Can you work these out from the model? Positions are in its coordinate system, mm. Coordinates: 2 decimals unless noted, no trailing zeros. Write each loop counter-clockwise with the first axis right and the second up, starting at its lowest first coordinate (ties: lowest second). Pieces come first, ordered by that corner, then holes. Notation, with made-up numbers: (-29, 65) - (0, 65) arc R14 ccw to (0, 72) - close; hole circle Ø3 at (66, 59). An arc over 180 degrees is marked (long way). Use one line per item in the form item = value. Start each with the question number.
(1) If we section it at A-A on x = 3.5: Please give me the cut outline in (y, z) (3 decimals).
(2) If we section it at B-B on z = 1478: Please give me the cut outline in (x, y) (3 decimals), then the cut area to 3 significant figures.
(3) If I drill on probe 1 along Y at (x, z) = (-1, 101.5) (3 decimals); probe 2 along X at (y, z) = (10.5, 1108.5), over which ranges is the centre line in solid material (lowest first)? Write a range as from..to.
Autodesk Inventor part; units mm, degrees
ref_plane "Start Plane" through (0, 0, 0) normal (0, 0, 1) x (1, 0, 0)
ref_plane "End Plane" through (0, 0, 1700) normal (0, 0, 1) x (1, 0, 0)
ref_plane "YZ Plane" through (0, 0, 0) normal (1, 0, 0) x (0, 1, 0)
ref_plane "Start Plane" through (0, 0, 0) normal (0, 0, 1) x (1, 0, 0)
ref_plane "End Plane" through (0, 0, 1700) normal (0, 0, 1) x (1, 0, 0)
sketch "Sketch" plane through (0, 0, 0) normal (0, 0, 1) x (1, 0, 0)
  line L0 (-15.875, -9.525) -> (-15.875, 9.525)
  line L1 (-9.525, 15.875) -> (9.525, 15.875)
  line L2 (15.875, 9.525) -> (15.875, -9.525)
  line L3 (9.525, -15.875) -> (-9.525, -15.875)
  arc A0 (-15.875, -9.525) -> (-9.525, -15.875) centre (-9.525, -9.525) ccw
  arc A1 (-9.525, 15.875) -> (-15.875, 9.525) centre (-9.525, 9.525) ccw
  arc A2 (15.875, 9.525) -> (9.525, 15.875) centre (9.525, 9.525) ccw
  arc A3 (9.525, -15.875) -> (15.875, -9.525) centre (9.525, -9.525) ccw
  arc A4 (-9.525, 12.7) -> (-12.7, 9.525) centre (-9.525, 9.525) ccw
  line L4 (-9.525, 12.7) -> (9.525, 12.7)
  arc A5 (12.7, 9.525) -> (9.525, 12.7) centre (9.525, 9.525) ccw
  line L5 (12.7, 9.525) -> (12.7, -9.525)
  arc A6 (9.525, -12.7) -> (12.7, -9.525) centre (9.525, -9.525) ccw
  line L6 (9.525, -12.7) -> (-9.525, -12.7)
  arc A7 (-12.7, -9.525) -> (-9.525, -12.7) centre (-9.525, -9.525) ccw
  line L7 (-12.7, -9.525) -> (-12.7, 9.525)
  line L8 (0, 24.0662) -> (0, -24.0662) construction
  line L9 (-24.0662, 0) -> (24.0662, 0) construction
  dimension "d10" = 31.75
  dimension "d11" = 31.75
  dimension "d12" = 3.175
  dimension "d15" = 15.875
  dimension "d16" = 15.875
  dimension "d17" = 6.35
extrude "Body" add sketch "Sketch" along normal up to surface (1700 mm away) from surface at 0
sketch "Sketch3" plane through (0, 0, 0) normal (0, 0, 1) x (1, 0, 0)
  line L0 (0, 0) -> (10, 0)
ref_plane "Work Plane3" through (0, 0, 0) normal (0, -1, 0) x (1, 0, 0)
sketch "Sketch5" plane through (-15.875, 9.525, 0) normal (-1, 0, 0) x (0, 0, 1)
  line L0 (309.525, 3.175) -> (290.475, 3.175)
  arc A0 (312.7, 0) -> (309.525, 3.175) centre (309.525, 0) ccw
  line L1 (312.7, -19.05) -> (312.7, 0)
  arc A1 (309.525, -22.225) -> (312.7, -19.05) centre (309.525, -19.05) ccw
  line L2 (290.475, -22.225) -> (309.525, -22.225)
  arc A2 (287.3, -19.05) -> (290.475, -22.225) centre (290.475, -19.05) ccw
  line L3 (287.3, 0) -> (287.3, -19.05)
  arc A3 (290.475, 3.175) -> (287.3, 0) centre (290.475, 0) ccw
  line L4 (284.125, -19.05) -> (284.125, 0)
  arc A4 (284.125, -19.05) -> (290.475, -25.4) centre (290.475, -19.05) ccw
  line L5 (309.525, -25.4) -> (290.475, -25.4)
  arc A5 (309.525, -25.4) -> (315.875, -19.05) centre (309.525, -19.05) ccw
  line L6 (315.875, 0) -> (315.875, -19.05)
  arc A6 (315.875, 0) -> (309.525, 6.35) centre (309.525, 0) ccw
  line L7 (290.475, 6.35) -> (309.525, 6.35)
  arc A7 (290.475, 6.35) -> (284.125, 0) centre (290.475, 0) ccw
  circle A8 centre (293.65, -9.525) radius 4
  line L8 (300, -22.225) -> (300, 3.175)
  line L9 (293.65, -3.1741) -> (299.15, -6.3496)
  line L10 (299.15, -6.3496) -> (299.15, -12.7004)
  line L11 (299.15, -12.7004) -> (293.65, -15.8759)
  line L12 (293.65, -15.8759) -> (288.15, -12.7004)
  line L13 (288.15, -12.7004) -> (288.15, -6.3496)
  line L14 (288.15, -6.3496) -> (293.65, -3.1741)
  circle A9 centre (306.35, -9.525) radius 4
  line L15 (306.35, -3.1741) -> (300.85, -6.3496)
  line L16 (300.85, -6.3496) -> (300.85, -12.7004)
  line L17 (300.85, -12.7004) -> (306.35, -15.8759)
  line L18 (306.35, -15.8759) -> (311.85, -12.7004)
  line L19 (311.85, -12.7004) -> (311.85, -6.3496)
  line L20 (311.85, -6.3496) -> (306.35, -3.1741)
  line L21 (6.35, 3.175) -> (25.4, 3.175)
  arc A10 (28.575, 0) -> (25.4, 3.175) centre (25.4, 0) ccw
  line L22 (28.575, 0) -> (28.575, -19.05)
  arc A11 (25.4, -22.225) -> (28.575, -19.05) centre (25.4, -19.05) ccw
  line L23 (25.4, -22.225) -> (6.35, -22.225)
  arc A12 (3.175, -19.05) -> (6.35, -22.225) centre (6.35, -19.05) ccw
  line L24 (3.175, -19.05) -> (3.175, 0)
  arc A13 (6.35, 3.175) -> (3.175, 0) centre (6.35, 0) ccw
  line L25 (31.75, -19.05) -> (31.75, 0)
  arc A14 (31.75, 0) -> (25.4, 6.35) centre (25.4, 0) ccw
  line L26 (25.4, 6.35) -> (6.35, 6.35)
  arc A15 (6.35, 6.35) -> (0, 0) centre (6.35, 0) ccw
  line L27 (0, 0) -> (0, -19.05)
  arc A16 (0, -19.05) -> (6.35, -25.4) centre (6.35, -19.05) ccw
  line L28 (6.35, -25.4) -> (25.4, -25.4)
  arc A17 (25.4, -25.4) -> (31.75, -19.05) centre (25.4, -19.05) ccw
  circle A18 centre (9.525, -9.525) radius 4
  line L29 (15.875, -22.225) -> (15.875, 3.175)
  line L30 (9.525, -3.1741) -> (15.025, -6.3496)
  line L31 (15.025, -6.3496) -> (15.025, -12.7004)
  line L32 (15.025, -12.7004) -> (9.525, -15.8759)
  line L33 (9.525, -15.8759) -> (4.025, -12.7004)
  line L34 (4.025, -12.7004) -> (4.025, -6.3496)
  line L35 (4.025, -6.3496) -> (9.525, -3.1741)
  line L36 (27.725, -12.7004) -> (27.725, -6.3496)
  line L37 (16.725, -6.3496) -> (16.725, -12.7004)
  line L38 (16.725, -12.7004) -> (22.225, -15.8759)
  line L39 (22.225, -15.8759) -> (27.725, -12.7004)
  circle A19 centre (22.225, -9.525) radius 4
  line L40 (27.725, -6.3496) -> (22.225, -3.1741)
  line L41 (22.225, -3.1741) -> (16.725, -6.3496)
  point P0 (0, -9.525)
  point P1 (300, -9.525)
  point P2 (299.15, -9.525)
  point P3 (300.85, -9.525)
  point P4 (15.875, -9.525)
  point P5 (15.025, -9.525)
  point P6 (16.725, -9.525)
  dimension "d20" = 8
  dimension "d22" = 11
  dimension "d23" = 6.35
  dimension "d26" = 8
  dimension "d27" = 11
  dimension "d28" = 6.35
extrude "Extrusion2" cut sketch "Sketch5" against normal through all contours A8 | A9 | A18 | A19
ref_plane "Work Plane4" through (0, 0, 850) normal (0, 0, -1) x (-1, 0, 0)
mirror "Mirror1" about plane through (0, 0, 850) normal (0, 0, -1) of "Extrusion2"
sketch "Sketch4" plane through (0, 0, 0) normal (0, -1, 0) x (1, 0, 0)
  line L0 (-2, 0) -> (12, 0)
  line L1 (-2, 1700) -> (12, 1700)
  dimension "d19" = 1700
equation "\"d10\" = G_H"
equation "\"d11\" = G_W"
equation "\"d12\" = G_T"
equation "\"d15\" = 0.5 * d10"
equation "\"d16\" = 0.5 * d11"
equation "\"d17\" = G_IR"
equation "\"d3\" = G_L"
equation "\"G_W\" = 31.75"
equation "\"G_H\" = 31.75"
equation "\"G_T\" = 3.175"
equation "\"G_IR\" = 6.35"
equation "\"G_L\" = d19"
equation "\"G_OFFSET_START\" = 0"
equation "\"G_OFFSET_END\" = 0"
equation "\"d14\" = G_OFFSET_END + B_L"
equation "\"B_L\" = 1700"
properties part number "AISC HSS - (1 1/4x1 1/4x1/8) - 66.929" material "Steel, Mild"
Reported:
q1.outline = (-15.875, 0) - (-12.7, 0) - (-12.7, 1700) - (-15.875, 1700) - close; (12.7, 0) - (15.875, 0) - (15.875, 1700) - (12.7, 1700) - close
q2.outline = (-15.875, -9.525) arc R6.35 ccw to (-9.525, -15.875) - (9.525, -15.875) arc R6.35 ccw to (15.875, -9.525) - (15.875, 9.525) arc R6.35 ccw to (9.525, 15.875) - (-9.525, 15.875) arc R6.35 ccw to (-15.875, 9.525) - close; hole (-12.7, -9.525) arc R3.175 ccw to (-9.525, -12.7) - (9.525, -12.7) arc R3.175 ccw to (12.7, -9.525) - (12.7, 9.525) arc R3.175 ccw to (9.525, 12.7) - (-9.525, 12.7) arc R3.175 ccw to (-12.7, 9.525) - close
q2.area = 337 mm2
q3.probe_1 = -15.875..-12.7, 12.7..15.875
q3.probe_2 = -15.8..-12.55, 12.55..15.8
